Build history of the part. All positions in model axes, mm. Coordinates: 2 decimals unless noted, no trailing zeros. Write each loop counter-clockwise with the first axis right and the second up, starting at its lowest first coordinate (ties: lowest second). Pieces come first, ordered by that corner, then holes.
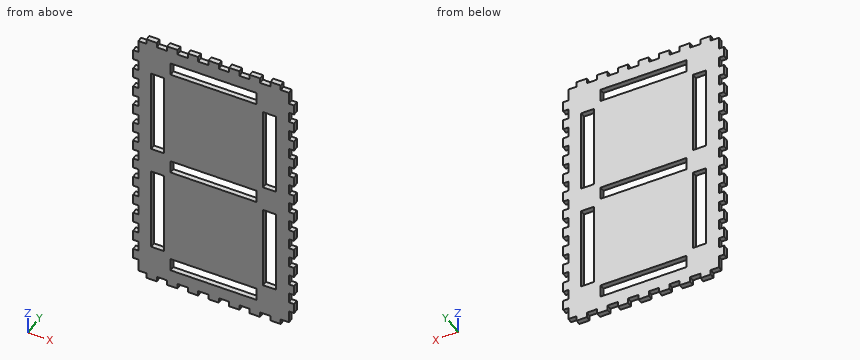
```python
from build123d import *

# Parameters (mm, degrees)
SKETCH3_W           = 15
SKETCH3_H           = 100
SKETCH3_W_2         = 100
SKETCH3_H_2         = 15
BOSS_EXTRUDE4_DEPTH = 6


with BuildPart() as part:
    # Sketch3 → Boss-Extrude4 (new body)
    with BuildSketch(Plane(origin=(0, 0, 0), x_dir=(1, 0, 0), z_dir=(0, 1, 0))):
        Polygon((-87.5, -152.5), (-78, -152.5), (-78, -158.5), (-66, -158.5), (-66, -152.5), (-54, -152.5), (-54, -158.5), (-42, -158.5), (-42, -152.5), (-30, -152.5), (-30, -158.5), (-18, -158.5), (-18, -152.5), (-6, -152.5), (-6, -158.5), (6, -158.5), (6, -152.5), (18, -152.5), (18, -158.5), (30, -158.5), (30, -152.5), (42, -152.5), (42, -158.5), (54, -158.5), (54, -152.5), (66, -152.5), (66, -158.5), (78, -158.5), (78, -152.5), (87.5, -152.5), (87.5, -138), (93.5, -138), (93.5, -126), (87.5, -126), (87.5, -114), (93.5, -114), (93.5, -102), (87.5, -102), (87.5, -90), (93.5, -90), (93.5, -78), (87.5, -78), (87.5, -66), (93.5, -66), (93.5, -54), (87.5, -54), (87.5, -42), (93.5, -42), (93.5, -30), (87.5, -30), (87.5, -18), (93.5, -18), (93.5, -6), (87.5, -6), (87.5, 6), (93.5, 6), (93.5, 18), (87.5, 18), (87.5, 30), (93.5, 30), (93.5, 42), (87.5, 42), (87.5, 54), (93.5, 54), (93.5, 66), (87.5, 66), (87.5, 78), (93.5, 78), (93.5, 90), (87.5, 90), (87.5, 102), (93.5, 102), (93.5, 114), (87.5, 114), (87.5, 126), (93.5, 126), (93.5, 138), (87.5, 138), (87.5, 152.5), (78, 152.5), (78, 158.5), (66, 158.5), (66, 152.5), (54, 152.5), (54, 158.5), (42, 158.5), (42, 152.5), (30, 152.5), (30, 158.5), (18, 158.5), (18, 152.5), (6, 152.5), (6, 158.5), (-6, 158.5), (-6, 152.5), (-18, 152.5), (-18, 158.5), (-30, 158.5), (-30, 152.5), (-42, 152.5), (-42, 158.5), (-54, 158.5), (-54, 152.5), (-66, 152.5), (-66, 158.5), (-78, 158.5), (-78, 152.5), (-87.5, 152.5), (-87.5, 138), (-93.5, 138), (-93.5, 126), (-87.5, 126), (-87.5, 114), (-93.5, 114), (-93.5, 102), (-87.5, 102), (-87.5, 90), (-93.5, 90), (-93.5, 78), (-87.5, 78), (-87.5, 66), (-93.5, 66), (-93.5, 54), (-87.5, 54), (-87.5, 42), (-93.5, 42), (-93.5, 30), (-87.5, 30), (-87.5, 18), (-93.5, 18), (-93.5, 6), (-87.5, 6), (-87.5, -6), (-93.5, -6), (-93.5, -18), (-87.5, -18), (-87.5, -30), (-93.5, -30), (-93.5, -42), (-87.5, -42), (-87.5, -54), (-93.5, -54), (-93.5, -66), (-87.5, -66), (-87.5, -78), (-93.5, -78), (-93.5, -90), (-87.5, -90), (-87.5, -102), (-93.5, -102), (-93.5, -114), (-87.5, -114), (-87.5, -126), (-93.5, -126), (-93.5, -138), (-87.5, -138), align=None)
        with Locations((-65, -65)):
            Rectangle(SKETCH3_W, SKETCH3_H, mode=Mode.SUBTRACT)
        with Locations((0, -130)):
            Rectangle(SKETCH3_W_2, SKETCH3_H_2, mode=Mode.SUBTRACT)
        Rectangle(SKETCH3_W_2, SKETCH3_H_2, mode=Mode.SUBTRACT)
        with Locations((65, -65)):
            Rectangle(SKETCH3_W, SKETCH3_H, mode=Mode.SUBTRACT)
        with Locations((-65, 65)):
            Rectangle(SKETCH3_W, SKETCH3_H, mode=Mode.SUBTRACT)
        with Locations((65, 65)):
            Rectangle(SKETCH3_W, SKETCH3_H, mode=Mode.SUBTRACT)
        with Locations((0, 130)):
            Rectangle(SKETCH3_W_2, SKETCH3_H_2, mode=Mode.SUBTRACT)
    extrude(amount=BOSS_EXTRUDE4_DEPTH)


solid = part.part
```
1. Saw through at C-C on x = -35.5. List the corners of the cut face in (y, z), plus the area to 3 significant figures.
Computed values:
outline: (0, -152.5) - (6, -152.5) - (6, -137.5) - (0, -137.5) - close; (0, -122.5) - (6, -122.5) - (6, -7.5) - (0, -7.5) - close; (0, 7.5) - (6, 7.5) - (6, 122.5) - (0, 122.5) - close; (0, 137.5) - (6, 137.5) - (6, 152.5) - (0, 152.5) - close
area: 1,560 mm2
2. Flat gauge pins, fed straight in: pin 1 (3 mm diameter, centred on y = 2.5, z = -25, fed in from +X); pin 2 (1.8 mm diameter, centred on y = 4, z = -156, fed in from -X); pin 3 (1.8 mm diameter, centred on x = -89, y = 2.5, fed in from +Z). Where does each tip first touch, or does it go through?
Computed values:
pin 1: stops at x = 87.5
pin 2: stops at x = -78
pin 3: stops at z = 138
3. Saw through at A-A on x = -61.5. List the corners of the cut face in (y, z), plus the area to 3 significant figures.
Computed values:
outline: (0, -152.5) - (6, -152.5) - (6, -115) - (0, -115) - close; (0, -15) - (6, -15) - (6, 15) - (0, 15) - close; (0, 115) - (6, 115) - (6, 152.5) - (0, 152.5) - close
area: 630 mm2
4. Saw through at B-B on z = -108. List the corners of the cut face in (x, y), plus the area to 3 significant figures.
Computed values:
outline: (-93.5, 0) - (-72.5, 0) - (-72.5, 6) - (-93.5, 6) - close; (-57.5, 0) - (57.5, 0) - (57.5, 6) - (-57.5, 6) - close; (72.5, 0) - (93.5, 0) - (93.5, 6) - (72.5, 6) - close
area: 942 mm2
5. Saw through at D-D on y = 4.9. State how many separate pieces and enclosed holes the cut face has, plus the area to 3 significant figures.
Computed values:
separate pieces: 1
enclosed holes: 7
area: 45,600 mm2
6. Probe line 1 along Z through (x, y) = (61, 4.45); line 2 along X through (y, z) = (1.6, -98.5); line 3 along Z through (x, y) = (44, 2.35). List the from-to ranges inside material, lowest first.
Computed values:
line 1: z = -152.5 to -115, -15 to 15, 115 to 152.5
line 2: x = -87.5 to -72.5, -57.5 to 57.5, 72.5 to 87.5
line 3: z = -158.5 to -137.5, -122.5 to -7.5, 7.5 to 122.5, 137.5 to 158.5
